from build123d import *

# Parameters (mm, degrees)
REVOLVE1_ANGLE = 358


with BuildPart() as part:
    # Sketch1 → Revolve1 (revolve)
    with BuildSketch(Plane.XY):
        with BuildLine():
            Line((-15, 0), (-24, 0))
            Line((-24, 0), (-24, 2.5))
            ThreePointArc((-24, 2.5), (-19.5, 7), (-15, 2.5))
            Line((-15, 2.5), (-15, 0))
        make_face()
        with BuildLine():
            Line((-16.5, 1.5), (-16.5, 2.5))
            ThreePointArc((-16.5, 2.5), (-19.5, 5.5), (-22.5, 2.5))
            Line((-22.5, 2.5), (-22.5, 1.5))
            Line((-22.5, 1.5), (-16.5, 1.5))
        make_face(mode=Mode.SUBTRACT)
    revolve(axis=Axis((0, 0, 0), (0, 1, 0)), revolution_arc=REVOLVE1_ANGLE)


solid = part.part
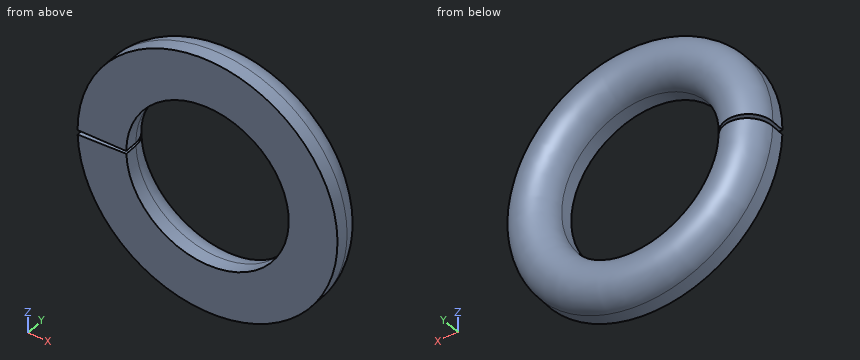
The listing builds one solid part. Answer for the finished solid, in the listing's coordinates (mm). Round coordinates to 2 decimals unless told otherwise and drop trailing zeros. Order: outer loops, then holes, each group sorted by start corner. A loop starts at its lowest first (then second) coordinate and runs counter-clockwise, first axis right, second up. Notation, with made-up numbers: (62, -12.75) -> (69, -12.75) arc R7 cw to (69, -5.75) -> close; hole circle Ø6 at (65.5, 30.5). An arc over 180 degrees is marked (long way). Put each result on its own line as item: value.
Q1. Consider line 1 along Z through (x, y) = (0, 1.95); line 2 along X through (y, z) = (5, 5.5); line 3 along Z through (x, y) = (-8, 3.75). Determine where each line is inside the solid, lowest interval first.
Results list:
line 1: -24 to -22.5, -16.5 to -15, 15 to 16.5, 22.5 to 24
line 2: -22.58 to -20.43, -16.97 to -14.77, 14.77 to 16.97, 20.43 to 22.58
line 3: -22.44 to -20.74, -14.74 to -12.9, 12.9 to 14.74, 20.74 to 22.44
Q2. Section A-A, the plane x = 0 is taken. Write down the section's boundary in (y, z), and give its area (3 significant figures).
Results list:
outline: (0, -24) -> (2.5, -24) arc R4.5 ccw to (2.5, -15) -> (0, -15) -> close; (0, 15) -> (2.5, 15) arc R4.5 ccw to (2.5, 24) -> (0, 24) -> close; hole (1.5, -22.5) -> (2.5, -22.5) arc R3 ccw to (2.5, -16.5) -> (1.5, -16.5) -> close; hole (1.5, 16.5) -> (2.5, 16.5) arc R3 ccw to (2.5, 22.5) -> (1.5, 22.5) -> close
area: 68.3 mm^2
Q3. Each of these flat-tipped pins is pushed along its axis until it touches: P1, Ø22.5, axis at x = 10, z = 7.5, coming from the +Y side; P2, Ø1.5, axis at y = 3, z = -4.5, coming from the -X side; P3, Ø4, axis at x = -13.5, y = 4.5, coming from the +Z side; P4, Ø1.5, axis at y = 2.5, z = 11, coming from the -X side. Where does it stop, or does it pass through?
Results list:
P1: y = 7
P2: x = -23.69
P3: z = 20.79
P4: x = -21.7
Q4. Section B-B, the plane y = 3.5 is taken. Write down the section's boundary in (x, z).
Results list:
outline: (-23.89, 0) -> (-22.33, 0) arc R22.33 cw (long way) to (-22.31, -0.78) -> (-23.87, -0.83) arc R23.89 ccw (long way) to start; (-16.67, 0) -> (-15.11, 0) arc R15.11 cw (long way) to (-15.1, -0.53) -> (-16.66, -0.58) arc R16.67 ccw (long way) to start
Q5. Section C-C, the plane z = -12 is taken. Count the separate pieces of the cut face and the enclosed holes in it, and give its area (3 significant figures).
Results list:
separate pieces: 2
enclosed holes: 2
area: 89.9 mm^2
